from build123d import *

# Parameters (mm, degrees)
SKETCH1_R           = 2
BOSS_EXTRUDE1_DEPTH = 9.525
FILLET1_R           = 2.54


with BuildPart() as part:
    # Sketch1 → Boss-Extrude1 (new body)
    with BuildSketch(Plane(origin=(0, 0, 0), x_dir=(1, 0, 0), z_dir=(0, 1, 0))):
        with BuildLine():
            Line((-12.7, -1.4125), (-12.7, -3))
            Line((-12.7, -3), (12.7, -3))
            Line((12.7, -3), (12.7, -1.4125))
            Line((12.7, -1.4125), (2.646666535, -1.4125))
            ThreePointArc((2.646666535, -1.4125), (0, 3), (-2.646666535, -1.4125))
            Line((-2.646666535, -1.4125), (-12.7, -1.4125))
        make_face()
        Circle(SKETCH1_R, mode=Mode.SUBTRACT)
    extrude(amount=BOSS_EXTRUDE1_DEPTH)

    # Fillet1
    fillet1_edges = [part.edges().sort_by_distance(p)[0] for p in [
        (-2.646666535, 4.7625, 1.4125),
        (2.646666535, 4.7625, 1.4125),
    ]]
    fillet(fillet1_edges, radius=FILLET1_R)


solid = part.part
Input: part model. Units: mm. Frame: model coordinates. A direction names the side the tool comes from. Round coordinates to 2 decimals unless told otherwise and drop trailing zeros. Loops run counter-clockwise (first coordinate to the right, second up) from the corner with the lowest first, then second, coordinate; pieces in that order, holes last. Notation, with made-up numbers: (3, -22) -> (48, -22) arc R12 ccw to (48, -14) -> close; hole circle Ø10 at (53.5, -38). An arc over 180 degrees is marked (long way). Answer as a JSON object with one key per item and string values. Group by question number.
1) Section query C-C on y = 1.25. Output: boundary loops of the cut face in (x, z), plus the area to 3 significant figures.
2) Draft query along X for faces 3 (the cylindrical face through (-3.84, 4.83, 0.86)), 4 (the cylindrical face through (0, 5, 2)), 5 (the flat face through (9, 5, 1.412)). Return one class per face: +X half, -X half, draft (parallel to the pull), parting line (faces both ways), or undercut.
3) Pin query (flat end, axial travel): pin 1 (3.5 mm diameter, centred on x = -8, y = 5.5, fed in from -Z); pin 2 (3 mm diameter, centred on y = 5, z = 0, fed in from -X); pin 3 (3 mm diameter, centred on x = 0, z = 0, fed in from -Y); pin 4 (1.5 mm diameter, centred on x = 2.5, y = 2, fed in from -Z). Return the tip coordinate at first contact, or that it passes through.
4) Section query B-B on z = -1.05. Output: boundary loops of the cut face in (x, y) (3 decimals), plus the area to 3 significant figures.
5) Section query D-D on x = 3.5. Output: boundary loops of the cut face in (y, z) (3 decimals).
6) Ray query, L1, parallel to X at y = 2.5, z = 0; L2, parallel to Z at x = 10, y = 3.5; L3, parallel to X at y = 7, z = 1.45. Return the intervals inside material, ascending.
7) Reachability of faces 1 (the cylindrical face through (0, 5, -3)), 2 (the flat face through (-9, 5, 1.412)) from +Z, -Z, +X, -X, +Y, -Y: full face, straight path, thin tool, end or side. Return the list, or none.
8) Section query A-A on x = 0. Output: boundary loops of the cut face in (y, z) (3 decimals).
Reply:
{
 "1": {"outline": "(-12.7, 1.41) -> (-5.42, 1.41) arc R2.54 cw to (-2.94, -0.61) arc R3 ccw to (2.94, -0.61) arc R2.54 cw to (5.42, 1.41) -> (12.7, 1.41) -> (12.7, 3) -> (-12.7, 3) -> close; hole circle Ø4 at (0, 0)", "area": "52.7 mm2"},
 "2": {"face 3": "-X half", "face 4": "undercut", "face 5": "draft"},
 "3": {"pin 1": "stops at z = 1.41", "pin 2": "stops at x = -12.7", "pin 3": "passes through", "pin 4": "stops at z = -2.44"},
 "4": {"outline": "(-2.81, 0) -> (-1.702, 0) -> (-1.702, 9.525) -> (-2.81, 9.525) -> close; (1.702, 0) -> (2.81, 0) -> (2.81, 9.525) -> (1.702, 9.525) -> close", "area": "21.1 mm2"},
 "5": {"outline": "(0, 0.531) -> (9.525, 0.531) -> (9.525, 3) -> (0, 3) -> close"},
 "6": {"L1": "x = -3.15 to -2, 2 to 3.15", "L2": "z = 1.41 to 3", "L3": "x = -12.7 to -1.38, 1.38 to 12.7"},
 "7": {"face 1": "-Z, +Y, -Y", "face 2": "-Z, -X, +Y, -Y"},
 "8": {"outline": "(0, -3) -> (9.525, -3) -> (9.525, -2) -> (0, -2) -> close; (0, 2) -> (9.525, 2) -> (9.525, 3) -> (0, 3) -> close"}
}
